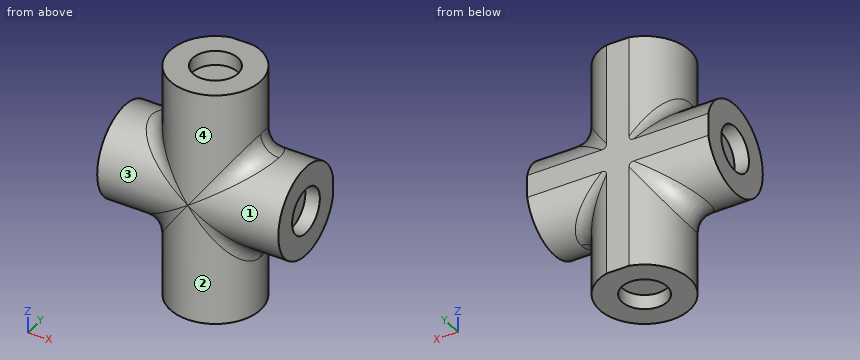
Autodesk Inventor part; units mm, degrees
ref_plane "YZ Plane" through (0, 0, 0) normal (1, 0, 0) x (0, 1, 0)
ref_plane "XZ Plane" through (0, 0, 0) normal (0, 1, 0) x (-1, 0, 0)
ref_plane "XY Plane" through (0, 0, 0) normal (0, 0, 1) x (1, 0, 0)
sketch "Sketch1" plane through (0, 0, 0) normal (0, 0, 1) x (1, 0, 0)
  circle A0 centre (0, 0) radius 2.5
  dimension "d0" = 5
extrude "Extrusion1" add sketch "Sketch1" along normal mid plane 13
sketch "Sketch2" plane through (0, 0, 6.5) normal (0, 0, 1) x (1, 0, 0)
  circle A0 centre (0, 0) radius 1.25
  dimension "d3" = 2.5
extrude "Extrusion2" cut sketch "Sketch2" against normal blind 0.8
mirror "Mirror1" about plane through (0, 0, 0) normal (0, 0, 1) of "Extrusion2"
sketch "Sketch3" plane through (0, 0, 0) normal (1, 0, 0) x (0, 1, 0)
  circle A0 centre (0, 0) radius 2.5
  dimension "d6" = 5
extrude "Extrusion3" add sketch "Sketch3" along normal mid plane 10
sketch "Sketch4" plane through (5, 0, 0) normal (1, 0, 0) x (0, 0, -1)
  circle A0 centre (0, 0) radius 1.25
  dimension "d9" = 2.5
extrude "Extrusion4" cut sketch "Sketch4" against normal blind 0.8
mirror "Mirror2" about plane through (0, 0, 0) normal (1, 0, 0) of "Extrusion4"
fillet "Fillet1" radius 1 6 edges at (1.7678, 1.7678, 1.7678) (-2.5, 0, 2.5) (1.7678, -1.7678, 1.7678) (1.7678, -1.7678, -1.7678) (1.7678, 1.7678, -1.7678) (-2.5, 0, -2.5)
sketch "Sketch5" plane through (0, 0, 6.5) normal (0, 0, 1) x (1, 0, 0)
  circle A0 centre (0, 0) radius 2.5
  line L0 (0, 2.5) -> (5.3723, 2.5)
  line L1 (5.3723, 2.5) -> (5.3723, 2.4205)
  line L2 (5.3723, 2.4205) -> (0, 2.4205)
  line L3 (0, 2.4205) -> (0, 2.5)
  line L4 (0, 2.5) -> (-5.4474, 2.5)
  line L5 (-5.4474, 2.5) -> (-5.4474, 2.4205)
  line L6 (-5.4474, 2.4205) -> (0, 2.4205)
  line L7 (0, 2.4205) -> (0, 2.5)
extrude "Extrusion5" cut sketch "Sketch5" against normal through all contours L2 L3 A0 | A0 L0 L1 L2 | L6 L5 L4 A0 | A0 L3 L6
ref_plane "Work Plane1" through (0, 0, 0) normal (0, 0, 1) x (1, 0, 0)
properties part number "_3DPrint"
Design review of the part built by this model. Coordinates are the model's own, in mm. Face numbers are marked on the shaded views. A direction names the side the tool comes from. Give positions to 0.01 mm unless a question says otherwise; leave off trailing zeros. Order: outer loops, then holes, each group sorted by start corner. A loop starts at its lowest first (then second) coordinate and runs counter-clockwise, first axis right, second up. Notation, with made-up numbers: (38.25, -33.75) - (63.25, -33.75) arc R33 cw to (63.25, -3.75) - close; hole circle Ø4 at (-21.5, -18). An arc over 180 degrees is marked (long way). Use a Markdown table: item, result. Add a question column.
(1) Add section A-A on z = -5.5. Give the boundary of the cut face in (x, y), then the cut area to 3 significant figures.
(2) Add section B-B on x = 4. Give the boundary of the cut face in (y, z), then the cut area to 3 significant figures.
(3) Clearance check with flat-ended pins moving along their axes: P1, Ø1.5, axis at x = 0, y = 0, coming from the -Z side; P2, Ø1.5, axis at x = 2, z = 3, coming from the -Y side; P3, Ø1, axis at x = -3.5, y = -2, coming from the -Z side. State where each tip first meets the part, or that it passes through.
(4) Wall thickness on probe 1 along Y at (x, z) = (0, 6.35); probe 2 along X at (y, z) = (-0.1, -0.5); probe 3 along Z at (x, y) = (3.75, -0.85): over which ranges is each line inside the solid? List them lowest first. Write a range as [from, to].
(5) Machinability: for the marked faces 1, 2, 3 and 4, which of the approach directions +Z, -Z, +X, -X, +Y, -Y give a long, thin tool a straight path to every point of the face, cutting with its end or side? Answer none if there is none.
Report:
| question | item | result |
|---|---|---|
| 1 | outline | (-0.63, 2.42) arc R2.5 ccw (long way) to (0.63, 2.42) - close |
| 1 | area | 19.6 mm² |
| 2 | outline | (2.42, -0.63) - (2.42, 0.63) arc R2.5 ccw (long way) to start |
| 2 | area | 19.6 mm² |
| 3 | P1 | stops at z = -5.7 |
| 3 | P2 | stops at y = -2.17 |
| 3 | P3 | stops at z = -2 |
| 4 | probe 1 | y = [-2.5, -1.25], [1.25, 2.42] |
| 4 | probe 2 | x = [-4.2, 4.2] |
| 4 | probe 3 | z = [-2.35, 2.35] |
| 5 | face 1 | +X |
| 5 | face 2 | -Z |
| 5 | face 3 | -X |
| 5 | face 4 | +Z |
